CAD build for the part. Positions are in the model's coordinates, mm. Round coordinates to 2 decimals unless told otherwise and drop trailing zeros. Loops run counter-clockwise (first coordinate to the right, second up) from the corner with the lowest first, then second, coordinate; pieces in that order, holes last. Notation, with made-up numbers: (26, 40) -> (32, 40) arc R25 cw to (32, 75) -> close; hole circle Ø4 at (-37.5, 44.25). An arc over 180 degrees is marked (long way). Answer as CSV lines item,"result".
```python
from build123d import *

# Parameters (mm, degrees)
SKETCH_1_R          = 27.5
EXTRUDE_1_DEPTH     = 2
FILLET_1_R          = 1
FILLET_2_R          = 1.3
SKETCH_4_W          = 16.091181195
SKETCH_4_H          = 8.262872831
SKETCH_4_W_2        = 19.931884343
SKETCH_4_W_3        = 14.487561678
SKETCH_4_H_2        = 5.890006991
SKETCH_4_W_4        = 16.715065691
SKETCH_4_H_3        = 8.177759915
SKETCH_4_W_5        = 10.105714663
SKETCH_4_H_4        = 26.066396506
SKETCH_4_W_6        = 5.661455371
SKETCH_4_H_5        = 27.456761526
CUT_EXTRUDE_1_DEPTH = 2


with BuildPart() as part:
    # 草图1 → 凸台-拉伸1 (new body)
    with BuildSketch(Plane.XY):
        Polygon((0, 0), (0, -4), (-1.45, -4), (-1.45, -7.2), (0, -7.2), (0, -10.4), (4.1, -10.4), (4.1, -7.2), (5.55, -7.2), (5.55, -4), (4.1, -4), (4.1, 0), (31.05, 0), (31.05, 5), (39.05, 5), (39.05, 0), (66, 0), (66, -4), (64.55, -4), (64.55, -7.2), (66, -7.2), (66, -10.4), (70.1, -10.4), (70.1, -7.2), (71.55, -7.2), (71.55, -4), (70.1, -4), (70.1, 0), (97.05, 0), (97.05, 5), (105.05, 5), (105.05, 0), (132, 0), (145.05, 0), (145.05, -63), (150.05, -63), (150.05, -71), (145.05, -71), (145.05, -97.95), (141.05, -97.95), (141.05, -96.490258022), (137.515203406, -96.490258022), (137.515203406, -97.95), (133.980406811, -97.95), (133.980406811, -102.05), (137.515203406, -102.05), (137.850237274, -103.470774067), (141.05, -103.509741978), (141.05, -102.05), (145.05, -102.05), (145.05, -129), (150.05, -129), (150.05, -137), (145.05, -137), (145.05, -200), (132, -200), (105.05, -200), (105.05, -205), (97.05, -205), (97.05, -200), (70.1, -200), (70.1, -196), (71.55, -196), (71.55, -192.8), (70.1, -192.8), (70.1, -189.6), (66, -189.6), (66, -192.8), (64.55, -192.8), (64.55, -196), (66, -196), (66, -200), (39.05, -200), (39.05, -205), (31.05, -205), (31.05, -200), (4.1, -200), (4.1, -196), (5.55, -196), (5.55, -192.8), (4.1, -192.8), (4.1, -189.6), (0, -189.6), (0, -192.8), (-1.45, -192.8), (-1.45, -196), (0, -196), (0, -200), (-26.95, -200), (-26.95, -205), (-34.95, -205), (-34.95, -200), (-61.9, -200), (-61.9, -196), (-60.45, -196), (-60.45, -192.8), (-61.9, -192.8), (-61.9, -189.6), (-66, -189.6), (-66, -192.8), (-67.45, -192.8), (-67.45, -196), (-66, -196), (-66, -200), (-92.95, -200), (-92.95, -205), (-100.95, -205), (-100.95, -200), (-127.9, -200), (-140.95, -200), (-140.95, -137), (-145.95, -137), (-145.95, -129), (-140.95, -129), (-140.95, -102.05), (-136.95, -102.05), (-136.95, -103.509741978), (-133.750237274, -103.470774067), (-133.415203406, -102.05), (-129.880406811, -102.05), (-129.880406811, -97.95), (-133.415203406, -97.95), (-133.415203406, -96.490258022), (-136.95, -96.490258022), (-136.95, -97.95), (-140.95, -97.95), (-140.95, -71), (-145.95, -71), (-145.95, -63), (-140.95, -63), (-140.95, 0), (-127.9, 0), (-100.95, 0), (-100.95, 5), (-92.95, 5), (-92.95, 0), (-66, 0), (-66, -4), (-67.45, -4), (-67.45, -7.2), (-66, -7.2), (-66, -10.4), (-61.9, -10.4), (-61.9, -7.2), (-60.45, -7.2), (-60.45, -4), (-61.9, -4), (-61.9, 0), (-34.95, 0), (-34.95, 5), (-26.95, 5), (-26.95, 0), align=None)
        with Locations((0, -100)):
            Circle(SKETCH_1_R, mode=Mode.SUBTRACT)
    extrude(amount=EXTRUDE_1_DEPTH)

    # 圆角1
    fillet_1_edges = [part.edges().sort_by_distance(p)[0] for p in [
        (-145.95, -63, 1),
        (-145.95, -71, 1),
        (-145.95, -129, 1),
        (-145.95, -137, 1),
    ]]
    fillet(fillet_1_edges, radius=FILLET_1_R)

    # 圆角2
    fillet_2_edges = [part.edges().sort_by_distance(p)[0] for p in [
        (39.05, 5, 1),
        (31.05, 5, 1),
        (-26.95, 5, 1),
        (-34.95, 5, 1),
        (-92.95, 5, 1),
        (-100.95, 5, 1),
        (-100.95, -205, 1),
        (-92.95, -205, 1),
        (-34.95, -205, 1),
        (-26.95, -205, 1),
        (31.05, -205, 1),
        (39.05, -205, 1),
        (97.05, -205, 1),
        (105.05, -205, 1),
        (150.05, -137, 1),
        (150.05, -129, 1),
        (150.05, -71, 1),
        (150.05, -63, 1),
        (105.05, 5, 1),
        (97.05, 5, 1),
    ]]
    fillet(fillet_2_edges, radius=FILLET_2_R)

    # 草图4 → 切除-拉伸1 (cut)
    with BuildSketch(Plane.XY.offset(2)):
        with Locations((-95.339833075, 6.131436416)):
            Rectangle(SKETCH_4_W, SKETCH_4_H)
        with Locations((100.859067665, 6.131436416)):
            Rectangle(SKETCH_4_W_2, SKETCH_4_H)
        with Locations((-97.37103045, -204.945003496)):
            Rectangle(SKETCH_4_W_3, SKETCH_4_H_2)
        with Locations((102.467476991, -206.088879958)):
            Rectangle(SKETCH_4_W_4, SKETCH_4_H_3)
        with Locations((-148.002857332, -124.681219337)):
            Rectangle(SKETCH_4_W_5, SKETCH_4_H_4)
        with Locations((149.880727686, -127.664492951)):
            Rectangle(SKETCH_4_W_6, SKETCH_4_H_5)
    extrude(amount=-CUT_EXTRUDE_1_DEPTH, mode=Mode.SUBTRACT)


solid = part.part
```
Q1. Slice it at C-C, the plane x = 61.5. Give the cut face in (y, z), and give its area (3 significant figures).
Results:
outline,"(-200, 0) -> (0, 0) -> (0, 2) -> (-200, 2) -> close"
area,"400 mm2"
Q2. Slice it at D-D, the plane y = -82.5. Give the cut face in (x, z).
Results:
outline,"(-140.95, 0) -> (-21.21, 0) -> (-21.21, 2) -> (-140.95, 2) -> close; (21.21, 0) -> (145.05, 0) -> (145.05, 2) -> (21.21, 2) -> close"
Q3. Probe L1, parallel to X at y = -195.5, z = 1.6; L2, parallel to X at y = -164, z = 0.95; L3, parallel to Y at x = -120.5, z = 1.7. List the from-to ranges inside material, lowest first. Write a range as [from, to].
Results:
L1,"[-140.95, -67.45], [-60.45, -1.45], [5.55, 64.55], [71.55, 145.05]"
L2,"[-140.95, 145.05]"
L3,"[-200, 0]"
Q4. Drop flat-ended pins along their axis: pin 1 Ø1.2 at (x, z) = (-66.5, 1) entering from +Y; pin 2 Ø1 at (y, z) = (-6, 1) entering from +X; pin 3 Ø0.6 at (x, z) = (-77, 0.5) entering from -Y; pin 4 Ø10 at (x, y) = (46, -70) entering from -Z. Give the stop position or say it passes through.
Results:
pin 1,"y = 0"
pin 2,"x = 145.05"
pin 3,"y = -200"
pin 4,"z = 0"
Q5. Slice it at B-B, the plane y = -166. Give the cut face in (x, z), and give its area (3 significant figures).
Results:
outline,"(-140.95, 0) -> (145.05, 0) -> (145.05, 2) -> (-140.95, 2) -> close"
area,"572 mm2"
Q6. Slice it at A-A, the plane y = -113. Give the cut face in (x, z).
Results:
outline,"(-140.95, 0) -> (-24.23, 0) -> (-24.23, 2) -> (-140.95, 2) -> close; (24.23, 0) -> (145.05, 0) -> (145.05, 2) -> (24.23, 2) -> close"
Q7. Two-plate mould, pull along Y, no slides. Class faces 1 (the flat face through (-29, -99, 0)), 2 (the cylindrical face through (-3.58, -72.734, 0.986)): pulls with the +Y half, pulls with the -Y half, needs draft (parallel to the pull), parting line crosses it, or undercut.
Results:
face 1,"needs draft"
face 2,"undercut"
